from build123d import *

# Parameters (mm, degrees)
SKETCH1_W           = 100
SKETCH1_H           = 7.5
BOSS_EXTRUDE1_DEPTH = 3
BOSS_EXTRUDE2_START = 50
SKETCH2_W           = 23
SKETCH2_H           = 7.5
BOSS_EXTRUDE2_DEPTH = 2
BOSS_EXTRUDE3_START = -50
SKETCH2_2_W         = 23
SKETCH2_2_H         = 7.5
BOSS_EXTRUDE3_DEPTH = 2
CUT_EXTRUDE1_START  = -50
SKETCH3_R           = 2.05
CUT_EXTRUDE1_DEPTH  = 103
CUT_EXTRUDE2_START  = 3
SKETCH4_R           = 2.05
CUT_EXTRUDE2_DEPTH  = 24


with BuildPart() as part:
    # Sketch1 → Boss-Extrude1 (new body)
    with BuildSketch(Plane.XY):
        Rectangle(SKETCH1_W, SKETCH1_H)
    extrude(amount=BOSS_EXTRUDE1_DEPTH)

    # Sketch2 → Boss-Extrude2 (add)
    with BuildSketch(Plane(origin=(0, 0, 0), x_dir=(0, 0, -1), z_dir=(1, 0, 0)).offset(BOSS_EXTRUDE2_START)):
        with Locations((8.5, 0)):
            Rectangle(SKETCH2_W, SKETCH2_H)
    extrude(amount=BOSS_EXTRUDE2_DEPTH)

    # Sketch2<2> → Boss-Extrude3 (add)
    with BuildSketch(Plane(origin=(0, 0, 0), x_dir=(0, 0, -1), z_dir=(1, 0, 0)).offset(BOSS_EXTRUDE3_START)):
        with Locations((8.5, 0)):
            Rectangle(SKETCH2_2_W, SKETCH2_2_H)
    extrude(amount=BOSS_EXTRUDE3_DEPTH)

    # Sketch3 → Cut-Extrude1 (cut, through all)
    with BuildSketch(Plane(origin=(0, 0, 0), x_dir=(0, 0, -1), z_dir=(1, 0, 0)).offset(CUT_EXTRUDE1_START)):
        with Locations((10, 0)):
            Circle(SKETCH3_R)
    extrude(amount=CUT_EXTRUDE1_DEPTH, mode=Mode.SUBTRACT)

    # Sketch4 → Cut-Extrude2 (cut, through all)
    with BuildSketch(Plane.XY.offset(CUT_EXTRUDE2_START)):
        Circle(SKETCH4_R)
    extrude(amount=-CUT_EXTRUDE2_DEPTH, mode=Mode.SUBTRACT)


solid = part.part
Source: CAD feature listing. Evaluate the final solid. Frame: model axes, mm. A direction names the side the tool comes from. Give positions to 0.01 mm unless a question says otherwise; leave off trailing zeros. Loops run counter-clockwise (first coordinate to the right, second up) from the corner with the lowest first, then second, coordinate; pieces in that order, holes last. Notation, with made-up numbers: (-9.75, 54) -> (6.25, 54) arc R14 cw to (6.25, 71) -> close; hole circle Ø2 at (62, 53). An arc over 180 degrees is marked (long way). Use a Markdown table: item, result. Add a question column.
1) Reachability of faces 4 (the face through (-7, -3.75, 2)), 5 (the face through (0.3, -2.4, 0)) from +Z, -Z, +X, -X, +Y, -Y: full face, straight path, thin tool, end or side. Return the list, or none.
2) First-contact query: pin 1 (4 mm diameter, centred on x = -10, y = -0.5, fed in from -Z). Flat tip, straight axial feed; report the tip coordinate or a pass-through.
3) Section query D-D, the plane x = 39. Return the cut outline in (y, z), then the cut area to 3 significant figures.
4) Pull-direction query (X, two-part tool) for faces 1 (the face through (-50, -2, -9)), 2 (the face through (-0.267, 2.033, 1.521)), 3 (the face through (-7, 3.75, 2)); classes: +X half, -X half, draft (parallel to the pull), parting line (faces both ways), or undercut.
5) Section query C-C, the plane z = -5.25. Return the cut outline in (x, y).
6) Section query A-A, the plane y = 0. Return the cut outline in (x, z), then the cut area to 3 significant figures.
7) Section query B-B, the plane z = -10. Return the cut outline in (x, y), then the cut area to 3 significant figures.
8) Line query: line 1 along Y through (x, z) = (51.5, -10); line 2 along Z through (x, y) = (-48.45, 0); line 3 along X through (y, z) = (1, -1.5). Output: solid intervals per line, ascending. Write a range as [from, to].
Numbers:
| question | item | result |
|---|---|---|
| 1 | face 4 | +Z, -Z, +X, -X, -Y |
| 1 | face 5 | -Z, +Y, -Y |
| 2 | pin 1 | stops at z = 0 |
| 3 | outline | (-3.75, 0) -> (3.75, 0) -> (3.75, 3) -> (-3.75, 3) -> close |
| 3 | area | 22.5 mm2 |
| 4 | face 1 | -X half |
| 4 | face 2 | undercut |
| 4 | face 3 | draft |
| 5 | outline | (-50, -3.75) -> (-48, -3.75) -> (-48, 3.75) -> (-50, 3.75) -> close; (50, -3.75) -> (52, -3.75) -> (52, 3.75) -> (50, 3.75) -> close |
| 6 | outline | (-50, -20) -> (-48, -20) -> (-48, -12.05) -> (-50, -12.05) -> close; (-50, -7.95) -> (-48, -7.95) -> (-48, 0) -> (-2.05, 0) -> (-2.05, 3) -> (-50, 3) -> close; (2.05, 0) -> (50, 0) -> (50, -7.95) -> (52, -7.95) -> (52, 3) -> (2.05, 3) -> close; (50, -20) -> (52, -20) -> (52, -12.05) -> (50, -12.05) -> close |
| 6 | area | 357 mm2 |
| 7 | outline | (-50, -3.75) -> (-48, -3.75) -> (-48, -2.05) -> (-50, -2.05) -> close; (-50, 2.05) -> (-48, 2.05) -> (-48, 3.75) -> (-50, 3.75) -> close; (50, -3.75) -> (52, -3.75) -> (52, -2.05) -> (50, -2.05) -> close; (50, 2.05) -> (52, 2.05) -> (52, 3.75) -> (50, 3.75) -> close |
| 7 | area | 13.6 mm2 |
| 8 | line 1 | y = [-3.75, -2.05], [2.05, 3.75] |
| 8 | line 2 | z = [-20, -12.05], [-7.95, 3] |
| 8 | line 3 | x = [-50, -48], [50, 52] |
